Autodesk Inventor part; units mm, degrees
ref_plane "YZ Plane" through (0, 0, 0) normal (1, 0, 0) x (0, 1, 0)
ref_plane "XZ Plane" through (0, 0, 0) normal (0, 1, 0) x (-1, 0, 0)
ref_plane "XY Plane" through (0, 0, 0) normal (0, 0, 1) x (1, 0, 0)
sketch "スケッチ1" plane through (0, 0, 0) normal (0, 0, 1) x (1, 0, 0)
  circle A0 centre (0, 0) radius 3
  circle A1 centre (0, 0) radius 1.5005
  dimension "d0" = 6
  dimension "d1" = 3.001
extrude "押し出し1" add sketch "スケッチ1" along normal blind 73
sketch "スケッチ2" plane through (0, 0, 73) normal (0, 0, 1) x (1, 0, 0)
  circle A0 centre (0, 0) radius 1.5005
  circle A1 centre (0, 0) radius 1.5
  dimension "d4" = 3
extrude "押し出し2" add sketch "スケッチ2" against normal blind 73
hole "穴1" at (0, 0, 73) direction (0, 0, -1) diameter 3 depth 6 tip angle 118
hole "穴2" at (0, 0, 0) direction (0, 0, 1) diameter 3 depth 6 tip angle 118
properties part number "スペーサーm3-73　簡易筒型" material "アルミニウム 2014-T4"
Work out the finished part from the listing and answer in its coordinate system (mm). A direction names the side the tool comes from. Round coordinates to 2 decimals unless told otherwise and drop trailing zeros. Order: outer loops, then holes, each group sorted by start corner. A loop starts at its lowest first (then second) coordinate and runs counter-clockwise, first axis right, second up. Notation, with made-up numbers: M 61,-37 L 65,-37 A23 cw 65,-29 Z; hole C 75.25,32 d11. An arc over 180 degrees is marked long. Put each result on its own line as item: value. Start each with the question number.
Q1. Section B-B, the plane y = -2.1 is taken. Write down the section's boundary in (x, z), and give its area (3 significant figures).
Q2. Section A-A, the plane z = 9 is taken. Write down the section's boundary in (x, y).
Q3. A tool of negligible diameter and unlimited length cuts with its end or side. For faces 1 (the cylindrical face through (-0.07, 1.5, 69.96)), 2 (the flat face through (1.3, -1.3, 73)), 3 (the cylindrical face through (-0.07, -1.5, 3.04)), from which of +Z, -Z, +X, -X, +Y, -Y can it reach the whole face along a straight path? Write none if from no direction.
Q4. A flat-ended cylindrical pin translates along its axis: pin 1 (2.5 mm diameter, centred on x = 0, y = 0, fed in from +Z). Find the tip coordinate at first contact, or state that the pin passes through.
Q5. Straight lines are drawn through the part: L1, parallel to Y at x = 0, z = 69.4; L2, parallel to Y at x = 0.2, z = 26; L3, parallel to Y at x = 2.1, z = 61.5. For each, find the intervals that lie inside material, in ascending order. Write a range as [from, to].
Findings below:
1. outline: M -2.14,0 L 2.14,0 L 2.14,73 L -2.14,73 Z
1. area: 313 mm^2
2. outline: C 0,0 d6
3. face 1: +Z
3. face 2: +Z, +X, -X, +Y, -Y
3. face 3: -Z
4. pin 1: stops at z = 66.85
5. L1: y = [-3, -1.5], [1.5, 3]
5. L2: y = [-2.99, 2.99]
5. L3: y = [-2.14, 2.14]
